The model under review builds one solid part; all positions refer to its coordinate system, in mm. A direction names the side the tool comes from. Give positions to 0.01 mm unless a question says otherwise; leave off trailing zeros. Loops run counter-clockwise (first coordinate to the right, second up) from the corner with the lowest first, then second, coordinate; pieces in that order, holes last. Notation, with made-up numbers: M 38,87.25 L 87,87.25 A21 ccw 87,97.25 Z; hole C 73,-7.75 d3. An arc over 180 degrees is marked long. Return JSON: item names as keys, results as strings.
Autodesk Inventor part; units mm, degrees
ref_plane "YZ Plane" through (0, 0, 0) normal (1, 0, 0) x (0, 1, 0)
ref_plane "XZ Plane" through (0, 0, 0) normal (0, 1, 0) x (-1, 0, 0)
ref_plane "XY Plane" through (0, 0, 0) normal (0, 0, 1) x (1, 0, 0)
sketch "草图1" plane through (0, 0, 0) normal (0, 1, 0) x (-1, 0, 0)
  line L0 (2.95, -1.7032) -> (0, -3.4064)
  line L1 (0, -3.4064) -> (-2.95, -1.7032)
  line L2 (-2.95, -1.7032) -> (-2.95, 1.7032)
  line L3 (-2.95, 1.7032) -> (0, 3.4064)
  line L4 (0, 3.4064) -> (2.95, 1.7032)
  line L5 (2.95, 1.7032) -> (2.95, -1.7032)
  point P0 (0, 0)
  point P1 (0, 0)
  point P2 (2.95, 0)
extrude "拉伸1" add sketch "草图1" along normal blind 15
sketch "草图2" plane through (0, 15, 0) normal (0, 1, 0) x (1, 0, 0)
  circle A0 centre (0, 0) radius 1.95
  dimension "d3" = 3.9
extrude "拉伸2" add sketch "草图2" along normal blind 25
thread "螺纹1"
sketch "草图6" plane through (0, 0, 0) normal (0, -1, 0) x (1, 0, 0)
  circle A0 centre (0, 0) radius 2
  dimension "d22" = 4
extrude "拉伸6" add sketch "草图6" along normal blind 35
sketch "草图7" plane through (0, -35, 0) normal (0, -1, 0) x (1, 0, 0)
  line L0 (10.5, -1.5) -> (10.5, 1.5)
  line L1 (-10.5, 1.5) -> (-10.5, -1.5)
  line L2 (-10.5, -1.5) -> (10.5, 1.5) construction
  line L3 (10.5, -1.5) -> (-10.5, 1.5) construction
  line L4 (-1.5, 10.5) -> (1.5, 10.5)
  line L5 (1.5, -10.5) -> (-1.5, -10.5)
  line L6 (-1.5, 10.5) -> (1.5, -10.5) construction
  line L7 (1.5, 10.5) -> (-1.5, -10.5) construction
  line L8 (-1.5, 1.5) -> (-10.5, 1.5)
  line L9 (10.5, 1.5) -> (1.5, 1.5)
  line L10 (1.5, 10.5) -> (1.5, 1.5)
  line L11 (1.5, -1.5) -> (1.5, -10.5)
  line L12 (1.5, -1.5) -> (10.5, -1.5)
  line L13 (-10.5, -1.5) -> (-1.5, -1.5)
  line L14 (-1.5, -10.5) -> (-1.5, -1.5)
  line L15 (-1.5, 1.5) -> (-1.5, 10.5)
  point P0 (0, 0)
  dimension "d26" = 21
extrude "拉伸7" add sketch "草图7" along normal blind 2
sketch "草图8" plane through (0, -37, 0) normal (0, -1, 0) x (1, 0, 0)
  circle A0 centre (0, 0) radius 9.5 construction
  circle A1 centre (0, 9.5) radius 0.75
  circle A2 centre (-9.5, 0) radius 0.75
  circle A3 centre (0, -9.5) radius 0.75
  circle A4 centre (9.5, 0) radius 0.75
  dimension "d29" = 19
  dimension "d30" = 1.5
  dimension "d31" = 1.5
  dimension "d32" = 1.5
  dimension "d33" = 1.5
extrude "拉伸8" add sketch "草图8" along normal blind 5
properties part number "杆件"
1) The part is to be moulded in two halves that separate along X. For faces 1 (the face through (8.75, -39.47, -0.03)), 2 (the face through (0, -37, 0)), 3 (the face through (10.5, -36, 0)), 4 (the face through (-6, -36, 1.5)), say which applies: released by +X, released by -X, zero draft, split by the parting line, or undercut.
From the geometry:
{"face 1": "undercut", "face 2": "undercut", "face 3": "released by +X", "face 4": "zero draft"}
2) Consider section A-A on x = 9.5. Write out the cut boundary in (y, z).
From the geometry:
{"outline": "M -42,-0.75 L -37,-0.75 L -37,-1.5 L -35,-1.5 L -35,1.5 L -37,1.5 L -37,0.75 L -42,0.75 Z"}
3) Insertion check: pin 1 (10.5 mm diameter, centred on x = -3, z = 2.5, fed in from +Y); pin 2 (8 mm diameter, centred on x = -5, z = -5.5, fed in from -Y); pin 3 (1.6 mm diameter, centred on x = 7.5, y = -36, fed in from +Z); pin 4 (10 mm diameter, centred on y = 9.5, z = 6.5, fed in from -X). Each pin has a flat end and moves straight along its axis. Give the tip position at first contact, or say it passes through.
From the geometry:
{"pin 1": "y = 40", "pin 2": "y = -37", "pin 3": "z = 1.5", "pin 4": "x = -2.95"}
4) Consider section C-C on y = 6. Write out the cut boundary in (x, z).
From the geometry:
{"outline": "M -2.95,-1.7 L 0,-3.41 L 2.95,-1.7 L 2.95,1.7 L 0,3.41 L -2.95,1.7 Z"}
5) Tool access review of faces 5 (the face through (1.5, 7.4, 2.54)), 6 (the face through (2.95, 7, 0)), 7 (the face through (-1.45, 7.4, 2.57)), 8 (the face through (-0.098, -39.465, -10.244)), 9 (the face through (-1.437, 27.325, 1.318)): name each direction out of +Z, -Z, +X, -X, +Y, -Y from which nothing blocks a thin tool from reaching the whole face with its end or side.
From the geometry:
{"face 5": "+Z, +X, +Y", "face 6": "+Z, -Z, +X, +Y", "face 7": "+Z, -X, +Y", "face 8": "-Y", "face 9": "+Y"}
6) Consider section D-D on z = 9.5. Write out the cut boundary in (x, y).
From the geometry:
{"outline": "M -1.5,-37 L -0.75,-37 L -0.75,-42 L 0.75,-42 L 0.75,-37 L 1.5,-37 L 1.5,-35 L -1.5,-35 Z"}
7) Wall thickness on L1, parallel to Y at x = -2.5, z = -0.5; L2, parallel to Y at x = -0.75, z = 7.5; L3, parallel to Z at x = -0.75, y = 24: over which ranges is each line inside the solid? List them lowest first. Write a range as from..to.
From the geometry:
{"L1": "-37..-35, 0..15", "L2": "-37..-35", "L3": "-1.8..1.8"}
8) Consider section B-B on z = 0. Write out the cut boundary in (x, y), then the cut area to 3 significant figures.
From the geometry:
{"outline": "M -10.5,-37 L -10.25,-37 L -10.25,-42 L -8.75,-42 L -8.75,-37 L 8.75,-37 L 8.75,-42 L 10.25,-42 L 10.25,-37 L 10.5,-37 L 10.5,-35 L 2,-35 L 2,0 L 2.95,0 L 2.95,15 L 1.95,15 L 1.95,40 L -1.95,40 L -1.95,15 L -2.95,15 L -2.95,0 L -2,0 L -2,-35 L -10.5,-35 Z", "area": "383 mm²"}
